Here's the drawing with two shaded views (mm, measured from the low corner). I have some questions. Give positions to 0.01 mm unless a question says otherwise; leave off trailing zeros. Write each loop counter-clockwise with the first axis right and the second up, starting at its lowest first coordinate (ties: lowest second). Pieces come first, ordered by that corner, then holes. Notation, with made-up numbers: (4.25, 73) - (13.25, 73) arc R17 cw to (13.25, 97) - close; hole circle Ø7 at (2, 63). An arc over 180 degrees is marked (long way). Use one line per item in the form item = value.
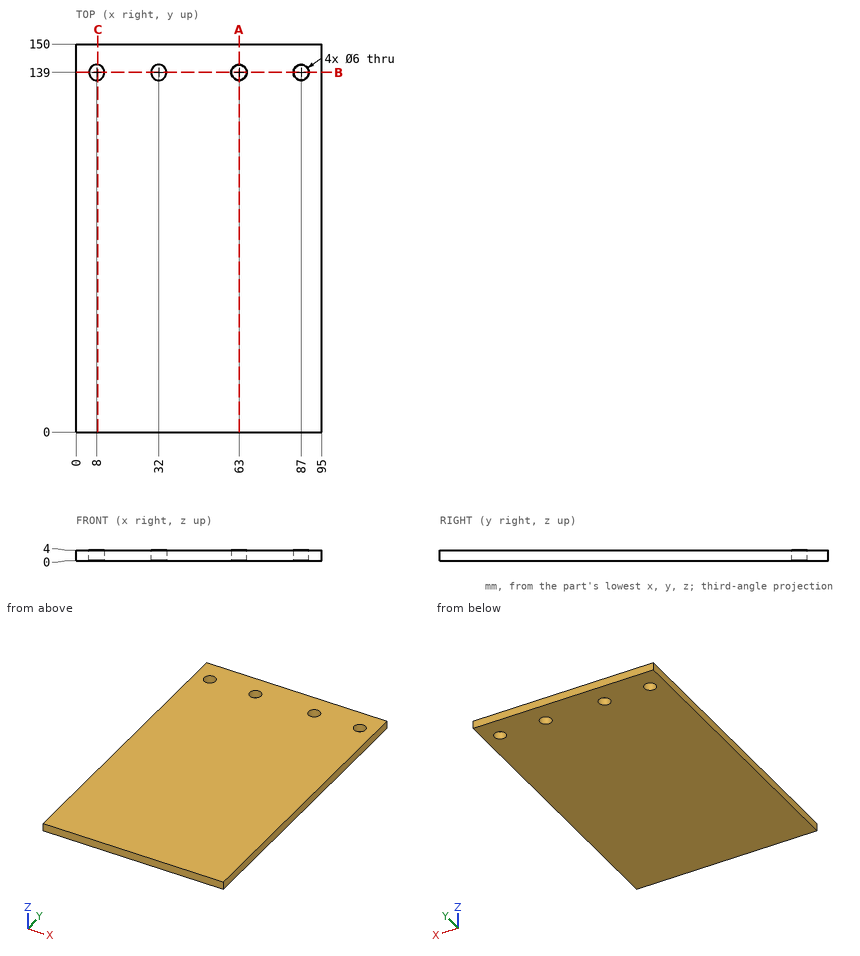
1. If I drill on line 1 (X direction, y = 139, z = 1.6); line 2 (Y direction, x = 8, z = 2.55), over which ranges is the centre line in solid material (lowest first)? Write a range as from..to.
Response values:
line_1 = 0..5, 11..29, 35..60, 66..84, 90..95
line_2 = 0..136, 142..150
2. For pin 1 (1 mm diameter, centred on x = 13.5, z = 1.5, fed in from -Y); pin 2 (5.5 mm diameter, centred on x = 32, y = 139, fed in from -Z), each with a flat end and sliding along its axis, tell me the tip position at first contact or that it passes through.
Response values:
pin_1 = 0
pin_2 = through
3. Imagine slicing it at C-C, the plane x = 8.5. List the corners of the cut face in (y, z) for me.
Response values:
outline = (0, 0) - (136.04, 0) - (136.04, 4) - (0, 4) - close; (141.96, 0) - (150, 0) - (150, 4) - (141.96, 4) - close
4. Imagine slicing it at B-B, the plane y = 139. List the corners of the cut face in (x, z) for me.
Response values:
outline = (0, 0) - (5, 0) - (5, 4) - (0, 4) - close; (11, 0) - (29, 0) - (29, 4) - (11, 4) - close; (35, 0) - (60, 0) - (60, 4) - (35, 4) - close; (66, 0) - (84, 0) - (84, 4) - (66, 4) - close; (90, 0) - (95, 0) - (95, 4) - (90, 4) - close
5. Imagine slicing it at A-A, the plane x = 63. List the corners of the cut face in (y, z) for me, and give its area (3 significant figures).
Response values:
outline = (0, 0) - (136, 0) - (136, 4) - (0, 4) - close; (142, 0) - (150, 0) - (150, 4) - (142, 4) - close
area = 576 mm²
